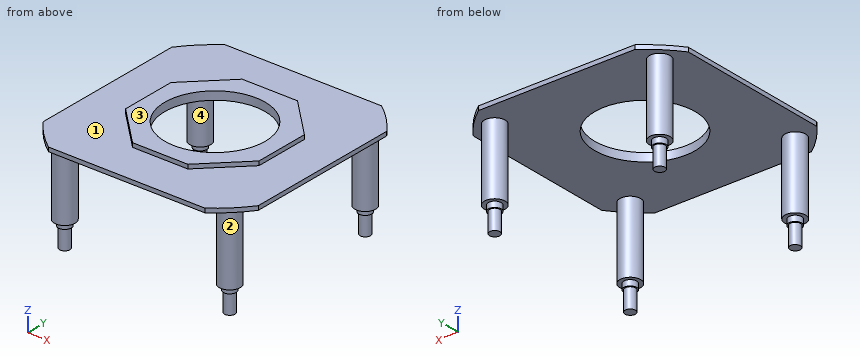
```python
from build123d import *

# Parameters (mm, degrees)
SKETCH1_W           = 203.947710216
SKETCH1_H           = 203.947710216
SKETCH1_R           = 38.5
BOSS_EXTRUDE1_DEPTH = 3.175
SKETCH1_3_R         = 38.5
BOSS_EXTRUDE2_DEPTH = 6.35
SKETCH2_R           = 8
BOSS_EXTRUDE3_DEPTH = 54.60355498
SKETCH3_R           = 5
BOSS_EXTRUDE4_DEPTH = 4.25
SKETCH4_R           = 4
BOSS_EXTRUDE5_DEPTH = 15
SKETCH6_W           = 203.947710216
SKETCH6_H           = 203.947710216
CUT_EXTRUDE1_DEPTH  = 15


with BuildPart() as part:
    # Sketch1 → Boss-Extrude1 (new body)
    with BuildSketch(Plane.XY):
        Rectangle(SKETCH1_W, SKETCH1_H)
        Polygon((51.2, 21.207734394), (21.207734394, 51.2), (-21.207734394, 51.2), (-51.2, 21.207734394), (-51.2, -21.207734394), (-21.207734394, -51.2), (21.207734394, -51.2), (51.2, -21.207734394), align=None, mode=Mode.SUBTRACT)
        Polygon((51.2, -21.207734394), (51.2, 21.207734394), (21.207734394, 51.2), (-21.207734394, 51.2), (-51.2, 21.207734394), (-51.2, -21.207734394), (-21.207734394, -51.2), (21.207734394, -51.2), align=None)
        Circle(SKETCH1_R, mode=Mode.SUBTRACT)
    extrude(amount=BOSS_EXTRUDE1_DEPTH)

    # Sketch1<3> → Boss-Extrude2 (add)
    with BuildSketch(Plane.XY):
        Polygon((51.2, -21.207734394), (51.2, 21.207734394), (21.207734394, 51.2), (-21.207734394, 51.2), (-51.2, 21.207734394), (-51.2, -21.207734394), (-21.207734394, -51.2), (21.207734394, -51.2), align=None)
        Circle(SKETCH1_3_R, mode=Mode.SUBTRACT)
    extrude(amount=BOSS_EXTRUDE2_DEPTH)

    # Sketch2 → Boss-Extrude3 (add)
    with BuildSketch(Plane(origin=(0, 0, 0), x_dir=(-1, 0, 0), z_dir=(0, 0, -1))):
        with Locations(Location((-63.286056916, 63.286056916, 0), (0, 0, 180))):
            Circle(SKETCH2_R)
    boss_extrude3 = extrude(amount=BOSS_EXTRUDE3_DEPTH)

    # Sketch3 → Boss-Extrude4 (add)
    with BuildSketch(Plane(origin=(0, 0, -54.60355498), x_dir=(-1, 0, 0), z_dir=(0, 0, -1))):
        with Locations((-63.286056916, 63.286056916)):
            Circle(SKETCH3_R)
    boss_extrude4 = extrude(amount=BOSS_EXTRUDE4_DEPTH)

    # Sketch4 → Boss-Extrude5 (add)
    with BuildSketch(Plane(origin=(0, 0, -58.85355498), x_dir=(-1, 0, 0), z_dir=(0, 0, -1))):
        with Locations((-63.286056916, 63.286056916)):
            Circle(SKETCH4_R)
    boss_extrude5 = extrude(amount=BOSS_EXTRUDE5_DEPTH)

    # Sketch-Pattern1: Boss-Extrude3, Boss-Extrude4, Boss-Extrude5 at 3 more places
    with Locations((-126.572114, 0, 0), (-126.572114, -126.572114, 0), (0, -126.572114, 0)):
        add(boss_extrude3)
        add(boss_extrude4)
        add(boss_extrude5)

    # Sketch6 → Cut-Extrude1 (cut)
    with BuildSketch(Plane(origin=(0, 0, 0), x_dir=(-1, 0, 0), z_dir=(0, 0, -1))):
        Rectangle(SKETCH6_W, SKETCH6_H)
        with BuildLine():
            ThreePointArc((-59.981247069, 82.5), (-72.124891681, 72.124891681), (-82.5, 59.981247069))
            Line((-82.5, 59.981247069), (-82.5, -59.981247069))
            ThreePointArc((-82.5, -59.981247069), (-72.124891681, -72.124891681), (-59.981247069, -82.5))
            Line((-59.981247069, -82.5), (59.981247069, -82.5))
            ThreePointArc((59.981247069, -82.5), (72.124891681, -72.124891681), (82.5, -59.981247069))
            Line((82.5, -59.981247069), (82.5, 59.981247069))
            ThreePointArc((82.5, 59.981247069), (72.124891681, 72.124891681), (59.981247069, 82.5))
            Line((59.981247069, 82.5), (-59.981247069, 82.5))
        make_face(mode=Mode.SUBTRACT)
    extrude(amount=-CUT_EXTRUDE1_DEPTH, mode=Mode.SUBTRACT)


solid = part.part
```
Design review of the part built by this model. Coordinates are the model's own, in mm. Face numbers are marked on the shaded views. A direction names the side the tool comes from. Coordinates: 2 decimals unless noted, no trailing zeros. Loops run counter-clockwise (first coordinate to the right, second up) from the corner with the lowest first, then second, coordinate; pieces in that order, holes last.
Q1. The part is to be moulded in two halves that separate along X. For the marked faces 1 and 2, say which applies: +X half, -X half, draft (parallel to the pull), parting line (faces both ways), or undercut.
Reported:
face 1: draft
face 2: undercut
Q2. We need section A-A on y = 0. State the section outline as (x, z) points (3 decimals), and give its area (3 significant figures).
Reported:
outline: (-82.5, 0) - (-38.5, 0) - (-38.5, 6.35) - (-51.2, 6.35) - (-51.2, 3.175) - (-82.5, 3.175) - close; (38.5, 0) - (82.5, 0) - (82.5, 3.175) - (51.2, 3.175) - (51.2, 6.35) - (38.5, 6.35) - close
area: 360 mm2
Q3. To check wall thickness, follow line 1 (X direction, y = -63, z = -20); line 2 (Y direction, x = 0, z = 5); line 3 (Y direction, x = 0, z = 2.25). State the ranges of each line that lie inside material, in increasing order.
Reported:
line 1: x = -71.28 to -55.29, 55.29 to 71.28
line 2: y = -51.2 to -38.5, 38.5 to 51.2
line 3: y = -82.5 to -38.5, 38.5 to 82.5
Q4. We need section D-D on z = -25. State the section outline as (x, y) points, and give its area (3 significant figures).
Reported:
outline: circle Ø16 at (-63.29, -63.29); circle Ø16 at (-63.29, 63.29); circle Ø16 at (63.29, -63.29); circle Ø16 at (63.29, 63.29)
area: 804 mm2
Q5. For pin 1 (5 mm diameter, centred on x = -47, y = -1.5, fed in from -Z); pin 2 (1 mm diameter, centred on x = -60.5, z = -25.5, fed in from +Y); pin 3 (2.5 mm diameter, centred on x = 10, z = 5, fed in from +Y), all flat-tipped, find the tip position at first contact; note any pin that passes through.
Reported:
pin 1: stops at z = 0
pin 2: stops at y = 70.95
pin 3: stops at y = 51.2
Q6. Tool access review of the marked faces 3 and 4: name each direction out of +Z, -Z, +X, -X, +Y, -Y from which nothing blocks a thin tool from reaching the whole face with its end or side.
Reported:
face 3: +Z, +X, -X, +Y, -Y
face 4: -Z
Q7. We need section C-C on z = -64. State the section outline as (x, y) points.
Reported:
outline: circle Ø8 at (-63.29, -63.29); circle Ø8 at (-63.29, 63.29); circle Ø8 at (63.29, -63.29); circle Ø8 at (63.29, 63.29)
